Source: three-view drawing plus pictorial views. Frame: mm from the lowest corner of the part. A direction names the side the tool comes from. Coordinates: 2 decimals unless noted, no trailing zeros. Write each loop counter-clockwise with the first axis right and the second up, starting at its lowest first coordinate (ties: lowest second). Pieces come first, ordered by that corner, then holes. Notation, with made-up numbers: (11, 12) - (54, 12) arc R19 ccw to (54, 22) - close; hole circle Ø8 at (-15, -12.75). An arc over 180 degrees is marked (long way). Answer as a JSON object with one key per item and string values. Group by question number.
Item 1: Section B-B on x = 9.25. Return loops of the section in (y, z).
Item 2: Section A-A on y = 5. Return loops of the section in (x, z) (3 decimals), and give its area (3 significant figures).
Item 3: Mould query, pull axis X, two halves, no side actions, for the marked faces 1, 2 and 3. Classes: pulls with the +X half, pulls with the -X half, needs draft (parallel to the pull), parting line crosses it, or undercut.
Item 4: Line query: line 1 along X through (y, z) = (1.25, 5); line 2 along Y through (x, z) = (8.75, 5); line 3 along Y through (x, z) = (5.5, 1). Output: solid intervals per line, ascending. Write a range as from..to.
Item 5: Section C-C on z = 3.75. Return loops of the section in (x, y) (3 decimals).
Item 6: Set-up query: the marked faces 4 and 5. Return all of +Z, -Z, +X, -X, +Y, -Y with unobstructed straight access to the full face (end or side cutting, diameter ignored); none if empty.
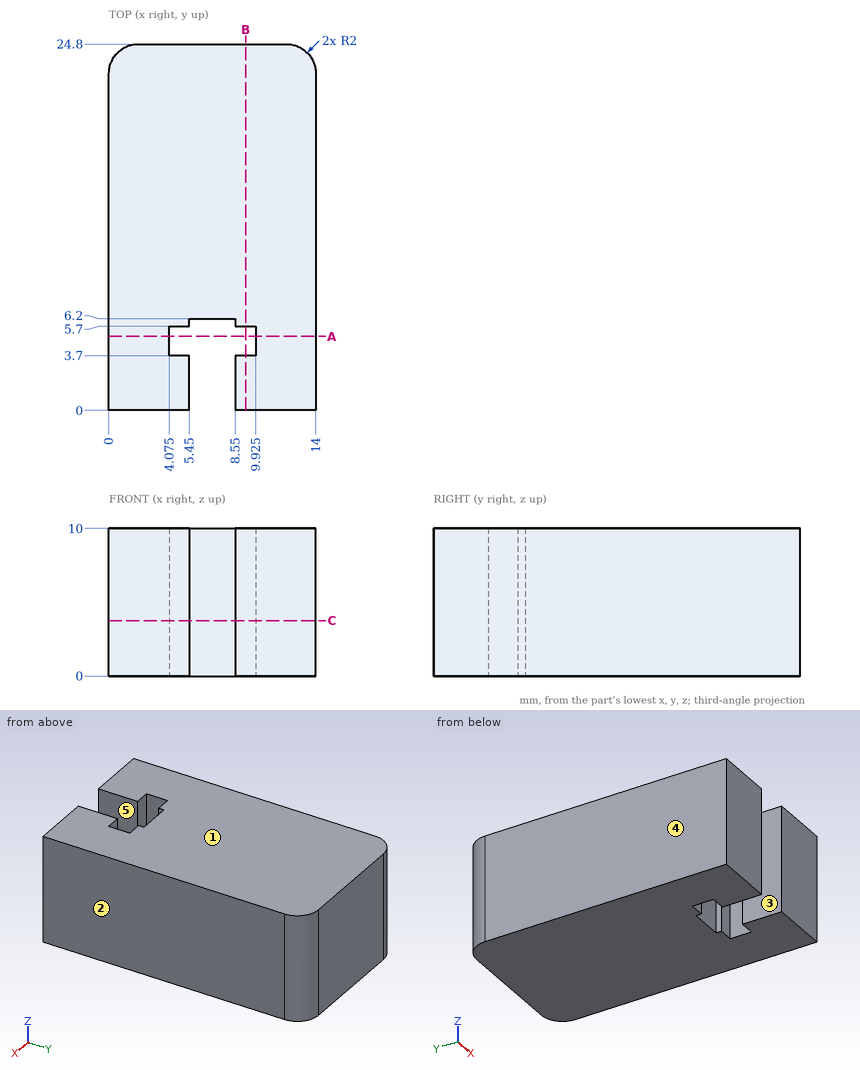
Checks:
{
 "1": {"outline": "(0, 0) - (3.7, 0) - (3.7, 10) - (0, 10) - close; (5.7, 0) - (24.8, 0) - (24.8, 10) - (5.7, 10) - close"},
 "2": {"outline": "(0, 0) - (4.075, 0) - (4.075, 10) - (0, 10) - close; (9.925, 0) - (14, 0) - (14, 10) - (9.925, 10) - close", "area": "81.5 mm^2"},
 "3": {"face 1": "needs draft", "face 2": "pulls with the +X half", "face 3": "undercut"},
 "4": {"line 1": "0..5.45, 8.55..14", "line 2": "0..3.7, 5.7..24.8", "line 3": "6.2..24.8"},
 "5": {"outline": "(0, 0) - (5.45, 0) - (5.45, 3.7) - (4.075, 3.7) - (4.075, 5.7) - (5.45, 5.7) - (5.45, 6.2) - (8.55, 6.2) - (8.55, 5.7) - (9.925, 5.7) - (9.925, 3.7) - (8.55, 3.7) - (8.55, 0) - (14, 0) - (14, 22.8) arc R2 ccw to (12, 24.8) - (2, 24.8) arc R2 ccw to (0, 22.8) - close"},
 "6": {"face 4": "+Z, -Z, -X, +Y, -Y", "face 5": "+Z, -Z, -Y"}
}
